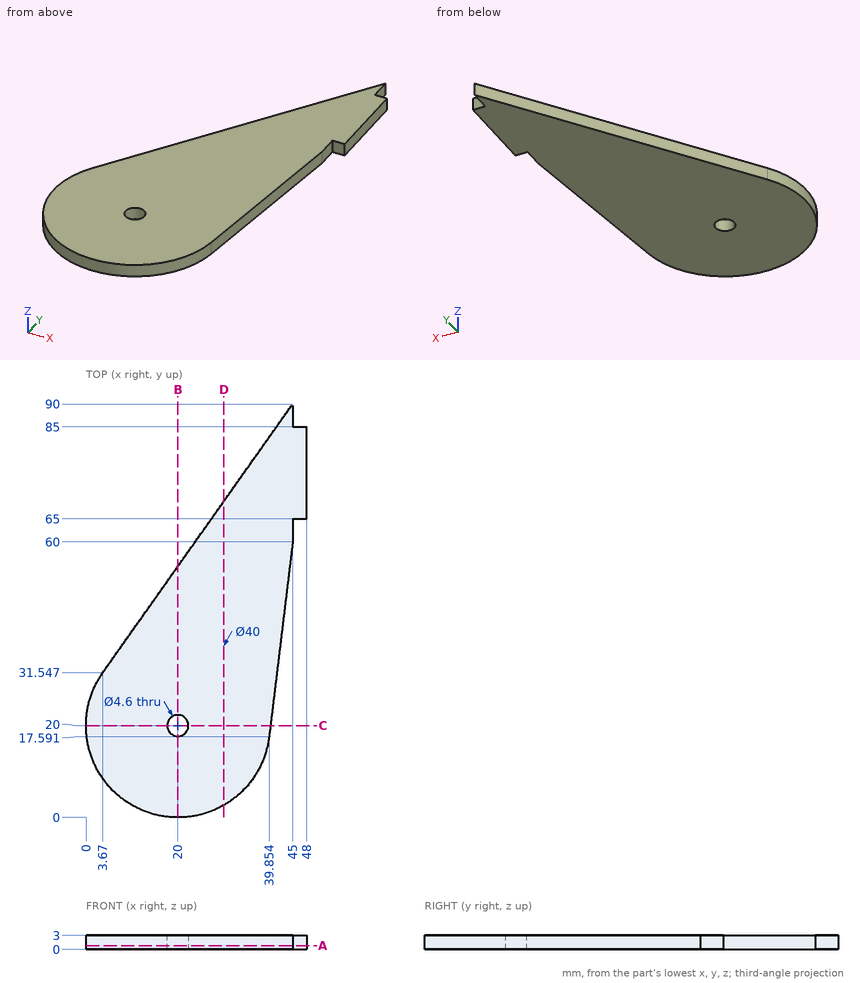
Check sheet for the drawn part. Datum: minimum x, y, z corner. Units: mm. Coordinates: 2 decimals unless noted, no trailing zeros. Loops run counter-clockwise (first coordinate to the right, second up) from the corner with the lowest first, then second, coordinate; pieces in that order, holes last. Notation, with made-up numbers: (81.25, 1) -> (127.25, 1) arc R20 cw to (127.25, 22) -> close; hole circle Ø6 at (19, 41). An arc over 180 degrees is marked (long way). Write each question's results on one line, items separated by ' | '.
Item 1: Section check B-B, the plane x = 20. Enter the section's corners in (y, z), plus the area to 3 significant figures.
Found:
outline: (0, 0) -> (17.7, 0) -> (17.7, 3) -> (0, 3) -> close; (22.3, 0) -> (54.64, 0) -> (54.64, 3) -> (22.3, 3) -> close | area: 150 mm2
Item 2: Section check D-D, the plane x = 30. Enter the section's corners in (y, z) (1 decimal), plus the area to 3 significant figures.
Found:
outline: (2.7, 0) -> (68.8, 0) -> (68.8, 3) -> (2.7, 3) -> close | area: 198 mm2
Item 3: Section check C-C, the plane y = 20. Enter the section's corners in (x, z).
Found:
outline: (0, 0) -> (17.7, 0) -> (17.7, 3) -> (0, 3) -> close; (22.3, 0) -> (40.15, 0) -> (40.15, 3) -> (22.3, 3) -> close
Item 4: Gauge pin test, flat ends, axial feed: pin 1 (1.5 mm diameter, centred on x = 47, z = 2, fed in from -Y); pin 2 (0.9 mm diameter, centred on x = 46, z = 1.5, fed in from +Y); pin 3 (3.5 mm diameter, centred on x = 20, y = 20, fed in from -Z). Record the tip position at first contact, or that the pin passes through.
Found:
pin 1: stops at y = 65 | pin 2: stops at y = 85 | pin 3: passes through
Item 5: Section check A-A, the plane z = 0.8. Enter the section's corners in (x, y) (1 decimal).
Found:
outline: (3.7, 31.5) arc R20 ccw (long way) to (39.9, 17.6) -> (45, 60) -> (45, 65) -> (48, 65) -> (48, 85) -> (45, 85) -> (45, 90) -> close; hole circle Ø4.6 at (20, 20)
Item 6: Material ranges on L1, parallel to Y at x = 18, z = 1.55 (1 decimal); L2, parallel to Y at x = 21.5, z = 0.4 (1 decimal); L3, parallel to Y at x = 35, z = 1.65 (1 decimal), recorded low to high.
Found:
L1: y = 0.1 to 18.9, 21.1 to 51.8 | L2: y = 0.1 to 18.3, 21.7 to 56.8 | L3: y = 6.8 to 75.9
